For this review, use the dimensioned drawing (mm, ordinates from the lowest corner) and the shaded views. Coordinates: 2 decimals unless noted, no trailing zeros. Order: outer loops, then holes, each group sorted by start corner. A loop starts at its lowest first (then second) coordinate and runs counter-clockwise, first axis right, second up. Notation, with made-up numbers: M 11,8 L 39,8 A30 ccw 39,34 Z; hole C 54,53.5 d7. An arc over 180 degrees is marked long. Answer as CSV lines item,"result". Start each with the question number.
Q1. Wall thickness on L1, parallel to X at y = 86.36, z = 50; L2, parallel to X at y = 45, z = 14; L3, parallel to X at y = 28, z = 71: over which ranges is each line inside the solid? List them lowest first. Write a range as [from, to].
Q2. Consider section C-C on z = 61. Write out the cut boundary in (x, y), and give its area (3 significant figures).
Q3. Consider section B-B on y = 89. Write out the cut boundary in (x, z).
Q4. For P1, Ø1, axis at y = 111.5, z = 46, coming from the -X side; P2, Ø7, axis at x = 32, y = 2.5, coming from the +Z side (1 decimal); P3, Ø22.5, axis at x = 5.5, z = 26.5, coming from the -Y side; P4, Ø2, axis at y = 19, z = 36, coming from the -X side, all flat-tipped, find the tip position at first contact; note any pin that passes through.
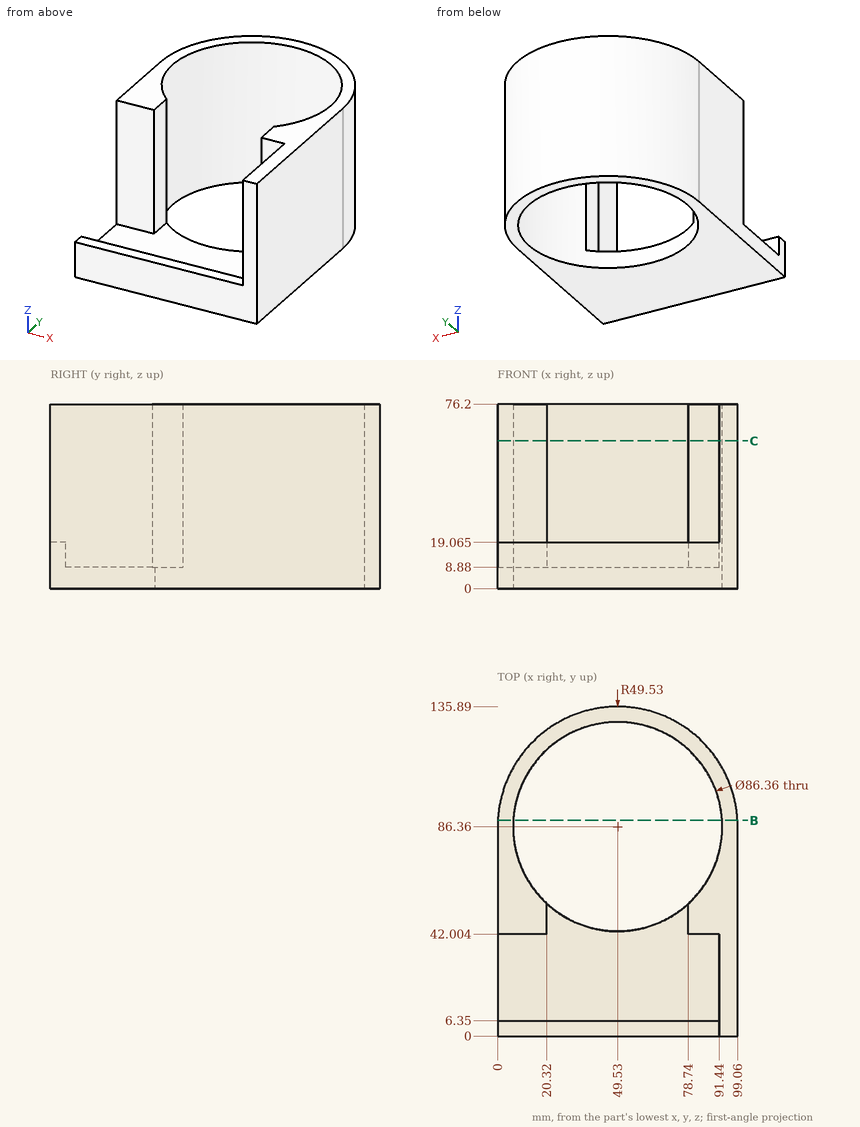
Evaluation:
1,L1,"x = [0, 6.35], [92.71, 99.06]"
1,L2,"x = [0, 20.32], [78.74, 99.06]"
1,L3,"x = [91.44, 99.06]"
2,outline,"M 0,42 L 20.32,42 L 20.32,54.56 A43.18 cw long 78.74,54.56 L 78.74,42 L 91.44,42 L 91.44,0 L 99.06,0 L 99.06,86.36 A49.53 ccw 0,86.36 Z"
2,area,"2,430 mm²"
3,outline,"M 0.07,0 L 6.43,0 L 6.43,76.2 L 0.07,76.2 Z; M 92.63,0 L 98.99,0 L 98.99,76.2 L 92.63,76.2 Z"
4,P1,"stops at x = 6.56"
4,P2,"stops at z = 19.1"
4,P3,"stops at y = 0"
4,P4,"stops at x = 91.44"
